Work out the finished part from the listing and answer in its coordinate system (mm). Give positions to 0.01 mm unless a question says otherwise; leave off trailing zeros. Order: outer loops, then holes, each group sorted by start corner. A loop starts at its lowest first (then second) coordinate and runs counter-clockwise, first axis right, second up. Notation, with made-up numbers: (88.5, 59) - (134.5, 59) arc R10 ccw to (134.5, 72) - close; hole circle Ø9 at (-19.5, 39). An arc over 180 degrees is marked (long way). Put each result on its own line as item: value.
```python
from build123d import *

# Parameters (mm, degrees)
SKETCH_1_W          = 22
SKETCH_1_H          = 370
EXTRUDE_1_DEPTH     = 5
SKETCH_2_R          = 1.55
CUT_EXTRUDE_1_DEPTH = 5
CUT_EXTRUDE_2_DEPTH = 5


with BuildPart() as part:
    # 草图1 → 凸台-拉伸1 (new body)
    with BuildSketch(Plane(origin=(0, 0, 0), x_dir=(1, 0, 0), z_dir=(0, 1, 0))):
        Rectangle(SKETCH_1_W, SKETCH_1_H)
    extrude(amount=EXTRUDE_1_DEPTH)

    # 草图2 → 切除-拉伸1 (cut)
    with BuildSketch(Plane(origin=(0, 5, 0), x_dir=(1, 0, 0), z_dir=(0, 1, 0))):
        with Locations(Location((0, 0, 0), (0, 0, 270))):
            Circle(SKETCH_2_R)
        with Locations(Location((0, 50, 0), (0, 0, 270))):
            Circle(SKETCH_2_R)
        with Locations(Location((0, 100, 0), (0, 0, 270))):
            Circle(SKETCH_2_R)
        with Locations(Location((0, 150, 0), (0, 0, 270))):
            Circle(SKETCH_2_R)
        with Locations(Location((0, -150, 0), (0, 0, 90))):
            Circle(SKETCH_2_R)
        with Locations(Location((0, -100, 0), (0, 0, 90))):
            Circle(SKETCH_2_R)
        with Locations(Location((0, -50, 0), (0, 0, 90))):
            Circle(SKETCH_2_R)
    extrude(amount=-CUT_EXTRUDE_1_DEPTH, mode=Mode.SUBTRACT)

    # 草图3 → 切除-拉伸2 (cut)
    with BuildSketch(Plane(origin=(0, 5, 0), x_dir=(1, 0, 0), z_dir=(0, 1, 0))):
        with BuildLine():
            Line((-5, 63), (-5, 87))
            ThreePointArc((-5, 87), (-4.121320344, 89.121320344), (-2, 90))
            Line((-2, 90), (2, 90))
            ThreePointArc((2, 90), (4.121320344, 89.121320344), (5, 87))
            Line((5, 87), (5, 63))
            ThreePointArc((5, 63), (4.121320344, 60.878679656), (2, 60))
            Line((2, 60), (-2, 60))
            ThreePointArc((-2, 60), (-4.121320344, 60.878679656), (-5, 63))
        make_face()
        with BuildLine():
            Line((-2, 110), (2, 110))
            ThreePointArc((2, 110), (4.121320344, 110.878679656), (5, 113))
            Line((5, 113), (5, 137))
            ThreePointArc((5, 137), (4.121320344, 139.121320344), (2, 140))
            Line((2, 140), (-2, 140))
            ThreePointArc((-2, 140), (-4.121320344, 139.121320344), (-5, 137))
            Line((-5, 137), (-5, 113))
            ThreePointArc((-5, 113), (-4.121320344, 110.878679656), (-2, 110))
        make_face()
        with BuildLine():
            Line((-5, 13), (-5, 37))
            ThreePointArc((-5, 37), (-4.121320344, 39.121320344), (-2, 40))
            Line((-2, 40), (2, 40))
            ThreePointArc((2, 40), (4.121320344, 39.121320344), (5, 37))
            Line((5, 37), (5, 13))
            ThreePointArc((5, 13), (4.121320344, 10.878679656), (2, 10))
            Line((2, 10), (-2, 10))
            ThreePointArc((-2, 10), (-4.121320344, 10.878679656), (-5, 13))
        make_face()
        with BuildLine():
            Line((-5, -37), (-5, -13))
            ThreePointArc((-5, -13), (-4.121320344, -10.878679656), (-2, -10))
            Line((-2, -10), (2, -10))
            ThreePointArc((2, -10), (4.121320344, -10.878679656), (5, -13))
            Line((5, -13), (5, -37))
            ThreePointArc((5, -37), (4.121320344, -39.121320344), (2, -40))
            Line((2, -40), (-2, -40))
            ThreePointArc((-2, -40), (-4.121320344, -39.121320344), (-5, -37))
        make_face()
        with BuildLine():
            Line((-5, -87), (-5, -63))
            ThreePointArc((-5, -63), (-4.121320344, -60.878679656), (-2, -60))
            Line((-2, -60), (2, -60))
            ThreePointArc((2, -60), (4.121320344, -60.878679656), (5, -63))
            Line((5, -63), (5, -87))
            ThreePointArc((5, -87), (4.121320344, -89.121320344), (2, -90))
            Line((2, -90), (-2, -90))
            ThreePointArc((-2, -90), (-4.121320344, -89.121320344), (-5, -87))
        make_face()
        with BuildLine():
            Line((-5, -137), (-5, -113))
            ThreePointArc((-5, -113), (-4.121320344, -110.878679656), (-2, -110))
            Line((-2, -110), (2, -110))
            ThreePointArc((2, -110), (4.121320344, -110.878679656), (5, -113))
            Line((5, -113), (5, -137))
            ThreePointArc((5, -137), (4.121320344, -139.121320344), (2, -140))
            Line((2, -140), (-2, -140))
            ThreePointArc((-2, -140), (-4.121320344, -139.121320344), (-5, -137))
        make_face()
    extrude(amount=-CUT_EXTRUDE_2_DEPTH, mode=Mode.SUBTRACT)


solid = part.part
```
(1) Section A-A, the plane z = -126 is taken. Write down the section's boundary in (x, y).
Geometry check:
outline: (-11, 0) - (-5, 0) - (-5, 5) - (-11, 5) - close; (5, 0) - (11, 0) - (11, 5) - (5, 5) - close
(2) Section B-B, the plane y = 2.9 is taken. Count the separate pieces of the cut face and the enclosed holes in it, then the cut area to 3 significant figures.
Geometry check:
separate pieces: 1
enclosed holes: 13
area: 6,330 mm²
(3) Straight lines are drawn through the part: line 1 (X direction, y = 2.6, z = 100); line 2 (X direction, y = 1.45, z = -62.5). For each, find the intervals that lie inside material, in ascending order.
Geometry check:
line 1: x = -11 to -1.55, 1.55 to 11
line 2: x = -11 to -4.96, 4.96 to 11
